Verification items for the finished model (mm, model axes). A direction names the side the tool comes from. Round coordinates to 2 decimals unless told otherwise and drop trailing zeros. Loops run counter-clockwise (first coordinate to the right, second up) from the corner with the lowest first, then second, coordinate; pieces in that order, holes last. Notation, with made-up numbers: M -33,27 L -20,27 A32 cw -20,56 Z; hole C 36.25,-3.5 d9. An arc over 180 degrees is marked long. Answer as CSV lines item,"result".
```python
from build123d import *

# Parameters (mm, degrees)
SALIENTE_EXTRUIR1_DEPTH = 200
CROQUIS3_R              = 2.05
CORTAR_EXTRUIR1_DEPTH   = 2.1
CROQUIS4_R              = 2.05
CORTAR_EXTRUIR2_DEPTH   = 2.1


with BuildPart() as part:
    # Croquis2 → Saliente-Extruir1 (new body)
    with BuildSketch(Plane.XY):
        Polygon((0, 0), (146.881, 0), (146.881, 99.2), (151.881, 99.2), (151.881, -5), (0, -5), align=None)
    extrude(amount=SALIENTE_EXTRUIR1_DEPTH)

    # Croquis3 → Cortar-Extruir1 (cut)
    with BuildSketch(Plane(origin=(0, 0, 0), x_dir=(1, 0, 0), z_dir=(0, 1, 0))):
        with Locations(Location((5, -195.5, 0), (0, 0, 270))):
            Circle(CROQUIS3_R)
        with Locations(Location((136.881, -195.5, 0), (0, 0, 270))):
            Circle(CROQUIS3_R)
        with Locations(Location((136.881, -4.5, 0), (0, 0, 90))):
            Circle(CROQUIS3_R)
        with Locations(Location((5, -4.5, 0), (0, 0, 90))):
            Circle(CROQUIS3_R)
    extrude(amount=-CORTAR_EXTRUIR1_DEPTH, mode=Mode.SUBTRACT)

    # Croquis4 → Cortar-Extruir2 (cut)
    with BuildSketch(Plane.ZY.offset(-146.881)):
        with Locations((4.5, 15)):
            Circle(CROQUIS4_R)
        with Locations((4.5, 94.7)):
            Circle(CROQUIS4_R)
        with Locations(Location((195.5, 15, 0), (0, 0, 180))):
            Circle(CROQUIS4_R)
        with Locations(Location((195.5, 94.7, 0), (0, 0, 180))):
            Circle(CROQUIS4_R)
    extrude(amount=-CORTAR_EXTRUIR2_DEPTH, mode=Mode.SUBTRACT)


solid = part.part
```
1) Draft check along X on faces 1 (the flat face through (5, -2.1, 195)), 2 (the flat face through (0, -3, 99)), 3 (the flat face through (149, 99.2, 99)). Enter one of: +X half, -X half, draft (parallel to the pull), parting line (faces both ways), or undercut.
Here are the results:
face 1,"undercut"
face 2,"-X half"
face 3,"draft"
2) Section check C-C (y = 80). Record the cut outline in (x, z).
Here are the results:
outline,"M 146.88,0 L 151.88,0 L 151.88,200 L 146.88,200 Z"
3) Material ranges on probe 1 along X at (y, z) = (-0.5, 195.5); probe 2 along X at (y, z) = (-1, 4); probe 3 along Y at (x, z) = (148.2, 195.5), recorded low to high.
Here are the results:
probe 1,"x = 0 to 2.95, 7.05 to 134.83, 138.93 to 151.88"
probe 2,"x = 0 to 3.01, 6.99 to 134.89, 138.87 to 151.88"
probe 3,"y = -5 to 12.95, 17.05 to 92.65, 96.75 to 99.2"
4) Set-up check for faces 4 (the cylindrical face through (147.916, 13.753, 2.873)), 5 (the flat face through (137, -2.1, 5)), 6 (the flat face through (146.881, 49, 99)): record each of +Z, -Z, +X, -X, +Y, -Y from which the full face is reachable in a straight line by a thin tool's end or side.
Here are the results:
face 4,"-X"
face 5,"+Y"
face 6,"+Z, -Z, -X, +Y"
5) Section check B-B (x = 111.5). Record the cut outline in (y, z), plus the area to 3 significant figures.
Here are the results:
outline,"M -5,0 L 0,0 L 0,200 L -5,200 Z"
area,"1,000 mm^2"
6) Section check A-A (z = 73). Record the cut outline in (x, y), plus the area to 3 significant figures.
Here are the results:
outline,"M 0,-5 L 151.88,-5 L 151.88,99.2 L 146.88,99.2 L 146.88,0 L 0,0 Z"
area,"1,260 mm^2"
7) Go/stop test with flat-tipped pins: pin 1 (1 mm diameter, centred on y = 77.5, z = 93, fed in from -X); pin 2 (2 mm diameter, centred on x = 5.5, z = 196, fed in from +Y); pin 3 (6 mm diameter, centred on x = 47.5, z = 129, fed in from +Y). Record where each tip stops, or that it passes through.
Here are the results:
pin 1,"stops at x = 146.88"
pin 2,"stops at y = -2.1"
pin 3,"stops at y = 0"
